Part model, mm, in its own coordinate system. Face numbers are marked on the shaded views. A direction names the side the tool comes from. Give positions to 0.01 mm unless a question says otherwise; leave off trailing zeros. Loops run counter-clockwise (first coordinate to the right, second up) from the corner with the lowest first, then second, coordinate; pieces in that order, holes last. Notation, with made-up numbers: M 33.5,-38.5 L 73.5,-38.5 A19 cw 73.5,-30.5 Z; hole C 0,50.25 d11. An arc over 180 degrees is marked long. Put each result on its own line as item: value. Start each with the question number.
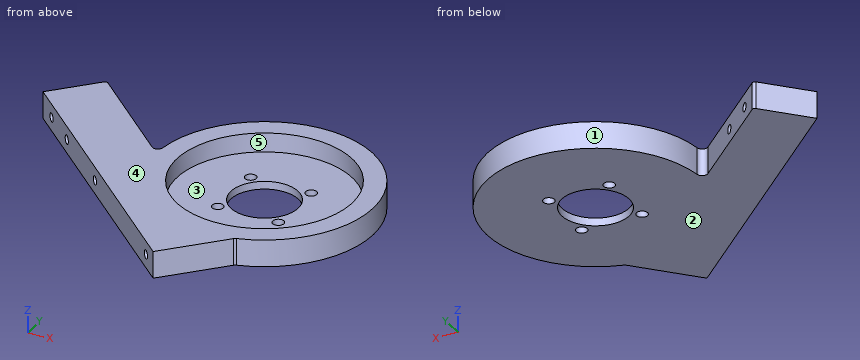
Autodesk Inventor part; units mm, degrees
ref_plane "Work Plane1" through (0, 0, 0) normal (0, 0, 1) x (1, 0, 0)
ref_plane "YZ Plane" through (0, 0, 0) normal (1, 0, 0) x (0, 1, 0)
ref_plane "XZ Plane" through (0, 0, 0) normal (0, 1, 0) x (-1, 0, 0)
ref_plane "Work Plane1" through (0, 0, 0) normal (0, 0, 1) x (1, 0, 0)
sketch "Sketch1" plane through (0, 0, 0) normal (0, 0, 1) x (1, 0, 0)
  arc A0 (-77.068, 33.987) -> (-78.4814, 33.9394) centre (-77.7509, 33.2565) ccw
  line L0 (-78.4814, 33.9394) -> (-92.9244, 18.4887)
  line L1 (-92.9244, 18.4887) -> (-9.2531, -59.7257)
  line L2 (-9.2531, -59.7257) -> (9.7389, -39.4086)
  arc A1 (10.6702, -38.8458) -> (9.7389, -39.4086) centre (11.2, -40.7744) ccw
  arc A2 (10.6702, -38.8458) -> (-40.1013, 3.8394) centre (0, 0) ccw
  line L3 (-43.4579, 2.5689) -> (-77.068, 33.987)
  circle A3 centre (33.3141, 1.123) radius 2.5
  circle A4 centre (1.123, -33.3141) radius 2.5
  circle A5 centre (0, 0) radius 21
  circle A6 centre (-1.123, 33.3141) radius 2.5
  circle A7 centre (-33.3141, -1.123) radius 2.5
  circle A8 centre (0, 0) radius 12.5
  circle A9 centre (0, -16) radius 2
  circle A10 centre (0, 16) radius 2
  circle A11 centre (-16, 0) radius 2
  circle A12 centre (16, 0) radius 2
  circle A13 centre (11.3137, 11.3137) radius 1.6
  circle A14 centre (-11.3137, -11.3137) radius 1.6
  circle A15 centre (-11.3137, 11.3137) radius 1.6
  circle A16 centre (11.3137, -11.3137) radius 1.6
  circle A17 centre (0, 0) radius 20.7
  circle A18 centre (0, 0) radius 40.2846
  line L4 (31.6375, -97.9493) -> (-99.8575, 24.9697)
  arc A19 (-43.4579, 2.5689) -> (-40.1013, 3.8394) centre (-42.0921, 4.03) ccw
  point P0 (0, 0)
  point P1 (-45.0314, -26.2807)
  point P2 (-23.1886, -46.699)
  point P3 (0, 0)
  point P4 (10.6702, -38.8458)
  point P5 (-40.1013, 3.8394)
  point P6 (0, 0)
extrude "Extrusion1" add sketch "Sketch1" along normal blind 10 contours L3 A19 A18 A1 L2 L1 L0 A0 | A2 A18 | A3 | A4 | A5 | A6 | A7 | A9 | A10 | A11 | A12 | A13 | A14 | A15 | A16 | A17
sketch "Sketch2" plane through (-77.068, 33.987, 10) normal (0.6828833, 0.7305275, 0) x (0.7305275, -0.6828833, 0)
  arc A0 (36.818, 70.5) -> (34.818, 72.5) centre (34.818, 70.5) ccw
  line L0 (-3.182, 72.5) -> (34.818, 72.5)
  arc A1 (-3.182, 72.5) -> (-5.182, 70.5) centre (-3.182, 70.5) ccw
  line L1 (-5.182, 2) -> (-5.182, 70.5)
  arc A2 (-5.182, 2) -> (-3.182, 0) centre (-3.182, 2) ccw
  line L2 (34.818, 0) -> (-3.182, 0)
  arc A3 (34.818, 0) -> (36.818, 2) centre (34.818, 2) ccw
  line L3 (36.818, 70.5) -> (36.818, 2)
  circle A4 centre (15.818, 36.25) radius 12.6
  circle A5 centre (31.818, 36.25) radius 2
  arc A6 (31.218, 2.9) -> (31.218, 7.1) centre (31.218, 5) ccw
  line L4 (0.418, 2.9) -> (31.218, 2.9)
  arc A7 (0.418, 7.1) -> (0.418, 2.9) centre (0.418, 5) ccw
  line L5 (31.218, 7.1) -> (0.418, 7.1)
  circle A8 centre (15.818, 20.25) radius 2
  arc A9 (0.418, 69.6) -> (0.418, 65.4) centre (0.418, 67.5) ccw
  line L6 (31.218, 69.6) -> (0.418, 69.6)
  arc A10 (31.218, 65.4) -> (31.218, 69.6) centre (31.218, 67.5) ccw
  line L7 (0.418, 65.4) -> (31.218, 65.4)
  circle A11 centre (15.818, 52.25) radius 2
  circle A12 centre (-0.182, 36.25) radius 2
  circle A13 centre (7.918, 67.5) radius 1.5706
  circle A14 centre (23.718, 67.5) radius 1.5706
  circle A15 centre (28.5459, 23.5221) radius 2
  circle A16 centre (3.09, 23.5221) radius 2
  circle A17 centre (3.09, 48.9779) radius 2
  circle A18 centre (28.5459, 48.9779) radius 2
  point P0 (79.5095, 10)
  point P1 (7.918, 5)
  point P2 (23.718, 5)
hole "Hole1" at (-71.2837, 28.58, 5) at (-59.7414, 17.7904, 5) direction (-0.6828833, -0.7305275, 0) diameter 3.242 end through all
sketch "Sketch9" plane through (0, 0, 10) normal (0, 0, 1) x (1, 0, 0)
  circle A0 centre (0, 0) radius 32.55
  dimension "d44" = 65.1
extrude "Extrusion4" cut sketch "Sketch9" against normal blind 7.1
sketch "Sketch11" plane through (-9.2531, -59.7257, 0) normal (-0.6828833, -0.7305275, 0) x (0.7305275, -0.6828833, 0)
  circle A0 centre (-60.5521, 5) radius 2.25
  circle A1 centre (-7.5, 5) radius 2.25
  point P0 (-34.026, 0)
hole "Hole7" at (-53.488, -18.3757, 5) at (-14.732, -54.604, 5) direction (0.6828833, 0.7305275, 0) diameter 3.242 depth 12.8 tip angle 118
sketch "Sketch12" plane through (0, 0, 2.9) normal (0, 0, 1) x (1, 0, 0)
  circle A0 centre (0, 0) radius 12.5
  circle A1 centre (0, -18) radius 2
  circle A2 centre (0, 18) radius 2
  circle A3 centre (-18, 0) radius 2
  circle A4 centre (18, 0) radius 2
  circle A5 centre (11.3137, 11.3137) radius 1.6
  circle A6 centre (-11.3137, -11.3137) radius 1.6
  circle A7 centre (-11.3137, 11.3137) radius 1.6
  circle A8 centre (11.3137, -11.3137) radius 1.6
  circle A9 centre (0, 0) radius 20.7
  point P0 (0, 0)
hole "Hole8" at (11.3137, 11.3137, 2.9) at (-11.3137, 11.3137, 2.9) at (-11.3137, -11.3137, 2.9) at (11.3137, -11.3137, 2.9) direction (0, 0, -1) diameter 4.2 depth 12.8 tip angle 118
properties part number "base frame voorkant 10 mm" material "Aluminum 6061"
1) Band-saw the part on A-A on y = -4. Give the cut face in (x, z), then the cut area to 3 significant figures.
2) Band-saw the part on D-D on y = 15.5. State how many separate pieces and enclosed holes the cut face has, then the cut area to 3 significant figures.
3) Which spindle directions (+Z, -Z, +X, -X, +Y, -Y) get a long thin tool onto all of the face, cutting with end or side? Do the marked faces 4 and 5. Say none if no direction does.
4) Band-saw the part on B-B on x = 0. Give the cut face in (y, z), then the cut area to 3 significant figures.
5) Pin check, flat tips, straight feed: pin 1 Ø19.5 at (x, y) = (11, -12.5) entering from +Z; pin 2 Ø1 at (y, z) = (-35.5, 6) entering from -X; pin 3 Ø3 at (y, z) = (1.5, 4.5) entering from -X. Stop position of each tip, or through.
6) Band-saw the part on C-C on z = 1.5. Give the cut face in (x, y).
7) Mould opens along Y. For the marked faces 1, 2 and 3 say: +Y half, -Y half, draft (parallel to the pull), parting line (faces both ways), or undercut.
8) Wall check: L1, parallel to Y at x = -11, z = 0.75; L2, parallel to X at y = 23, z = 8.5; L3, parallel to Z at x = -5, y = 26. Give the ranges that are in metal, low to high.
Evaluation:
1. outline: M -68.87,0 L -11.84,0 L -11.84,2.9 L -32.3,2.9 L -32.3,10 L -68.87,10 Z; M 11.84,0 L 40.09,0 L 40.09,10 L 32.3,10 L 32.3,2.9 L 11.84,2.9 Z
1. area: 562 mm2
2. separate pieces: 2
2. enclosed holes: 2
2. area: 639 mm2
3. face 4: +Z, +X, -X, +Y, -Y
3. face 5: +Z
4. outline: M -49.83,0 L -12.5,0 L -12.5,2.9 L -32.55,2.9 L -32.55,10 L -49.83,10 Z; M 12.5,0 L 40.28,0 L 40.28,10 L 32.55,10 L 32.55,2.9 L 12.5,2.9 Z
4. area: 366 mm2
5. pin 1: z = 2.9
5. pin 2: x = -35.7
5. pin 3: x = -76.36
6. outline: M -92.92,18.49 L -9.25,-59.73 L 9.74,-39.41 A2 cw 10.67,-38.85 A40.28 ccw long -40.1,3.84 A2 cw -43.46,2.57 L -77.07,33.99 A1 ccw -78.48,33.94 Z; hole C -11.31,-11.31 d4.2; hole C -11.31,11.31 d4.2; hole C 0,0 d25; hole C 11.31,-11.31 d4.2; hole C 11.31,11.31 d4.2
7. face 1: parting line
7. face 2: draft
7. face 3: undercut
8. L1: -58.09 to -13.39, -9.24 to -5.94, 5.94 to 9.24, 13.39 to 38.75
8. L2: -88.71 to -65.31, -33.07 to -23.03, 23.03 to 33.07
8. L3: 0 to 2.9
